```python
from build123d import *

# Parameters (mm, degrees)
BOSS_EXTRUDE1_DEPTH     = 250
BOSS_EXTRUDE2_DEPTH     = 50
SKETCH3_R               = 5
CUT_EXTRUDE1_DEPTH      = 319.801276513
FILLET1_R               = 10
MIRROR2_COPY_1_SKETCH_R = 5
MIRROR2_COPY_1_DEPTH    = 319.801276513
FILLET1_OF_MIRROR2_R    = 10
CUT_EXTRUDE2_DEPTH      = 282.035202699
FILLET2_R               = 25
CUT_EXTRUDE3_DEPTH      = 282.035202699
FILLET3_R               = 25
SKETCH6_R               = 5
CUT_EXTRUDE4_DEPTH      = 280.207367213
CUT_EXTRUDE5_DEPTH      = 170
FILLET4_R               = 10
FILLET5_R               = 25.875
FILLET6_R               = 10
BOSS_EXTRUDE3_DEPTH     = 30
SKETCH9_W               = 15.875
SKETCH9_H               = 40
BOSS_EXTRUDE4_DEPTH     = 140
FILLET7_R               = 25.875
FILLET8_R               = 10
SKETCH10_W              = 8.436021397
SKETCH10_H              = 40
CUT_EXTRUDE6_DEPTH      = 130
SKETCH11_R              = 5
CUT_EXTRUDE7_DEPTH      = 280.207367213


with BuildPart() as part:
    # Sketch1 → Boss-Extrude1 (new body)
    with BuildSketch(Plane.XY):
        Polygon((0, 0), (0, 110), (15.875, 110), (15.875, 0), (40, 0), (40, -70), (24.125, -70), (24.125, -15.875), (0, -15.875), align=None)
    extrude(amount=BOSS_EXTRUDE1_DEPTH)

    # Sketch2 → Boss-Extrude2 (add)
    with BuildSketch(Plane(origin=(0, 0, 0), x_dir=(-1, 0, 0), z_dir=(0, 0, -1))):
        Polygon((-32.0625, -70), (-82.0625, -70), (-82.0625, -77.9375), (17.9375, -77.9375), (17.9375, -70), align=None)
    boss_extrude2 = extrude(amount=-BOSS_EXTRUDE2_DEPTH)

    # Sketch3 → Cut-Extrude1 (cut, through all)
    with BuildSketch(Plane(origin=(0, -70, 0), x_dir=(1, 0, 0), z_dir=(0, 1, 0))):
        with Locations(Location((61.03125, -25, 0), (0, 0, 180))):
            Circle(SKETCH3_R)
    cut_extrude1 = extrude(amount=-CUT_EXTRUDE1_DEPTH, mode=Mode.SUBTRACT)

    # Mirror1: Cut-Extrude1 across plane
    add(cut_extrude1.mirror(Plane(origin=(32.0625, 0, 0), x_dir=(0, 0, 1), z_dir=(1, 0, 0))), mode=Mode.SUBTRACT)

    # Fillet1
    fillet1_edges = [part.edges().sort_by_distance(p)[0] for p in [
        (40, -70, 25),
        (24.125, -70, 25),
    ]]
    fillet(fillet1_edges, radius=FILLET1_R)

    # Mirror2: Boss-Extrude2, Cut-Extrude1 across plane
    add(boss_extrude2.mirror(Plane(origin=(0, 0, 125), x_dir=(1, 0, 0), z_dir=(0, 0, -1))))
    add(cut_extrude1.mirror(Plane(origin=(0, 0, 125), x_dir=(1, 0, 0), z_dir=(0, 0, -1))), mode=Mode.SUBTRACT)

    # Mirror2 copy 1 sketch → Mirror2 copy 1 (cut, through all)
    with BuildSketch(Plane(origin=(64.125, -70, 250), x_dir=(-1, 0, 0), z_dir=(0, 1, 0))):
        with Locations(Location((61.03125, -25, 0), (0, 0, 180))):
            Circle(MIRROR2_COPY_1_SKETCH_R)
    extrude(amount=-MIRROR2_COPY_1_DEPTH, mode=Mode.SUBTRACT)

    # Fillet1 of Mirror2
    fillet1_of_mirror2_edges = [part.edges().sort_by_distance(p)[0] for p in [
        (40, -70, 225),
        (24.125, -70, 225),
    ]]
    fillet(fillet1_of_mirror2_edges, radius=FILLET1_OF_MIRROR2_R)

    # Sketch4 → Cut-Extrude2 (cut, through all)
    with BuildSketch(Plane(origin=(15.875, 0, 0), x_dir=(0, 0, -1), z_dir=(1, 0, 0))):
        Polygon((0, 0), (-140, 0), (-140, 20), (-40, 20), (-40, 110), (0, 110), align=None)
    extrude(amount=-CUT_EXTRUDE2_DEPTH, mode=Mode.SUBTRACT)

    # Fillet2
    fillet2_edges = [part.edges().sort_by_distance(p)[0] for p in [
        (7.9375, 110, 40),
    ]]
    fillet(fillet2_edges, radius=FILLET2_R)

    # Sketch5 → Cut-Extrude3 (cut, through all)
    with BuildSketch(Plane(origin=(15.875, 0, 0), x_dir=(0, 0, -1), z_dir=(1, 0, 0))):
        Polygon((-250, 60), (-250, 110), (-200, 110), align=None)
    extrude(amount=-CUT_EXTRUDE3_DEPTH, mode=Mode.SUBTRACT)

    # Fillet3
    fillet3_edges = [part.edges().sort_by_distance(p)[0] for p in [
        (7.9375, 60, 250),
        (7.9375, 110, 200),
    ]]
    fillet(fillet3_edges, radius=FILLET3_R)

    # Sketch6 → Cut-Extrude4 (cut, through all)
    with BuildSketch(Plane(origin=(40, 0, 0), x_dir=(0, 0, -1), z_dir=(1, 0, 0))):
        with Locations((-65, 85)):
            Circle(SKETCH6_R)
        with Locations((-100, 85)):
            Circle(SKETCH6_R)
        with Locations((-128, 30)):
            Circle(SKETCH6_R)
        with Locations((-155, 20)):
            Circle(SKETCH6_R)
        with Locations(Location((-35, -25, 0), (0, 0, 90))):
            Circle(SKETCH6_R)
        with Locations(Location((-85, -25, 0), (0, 0, 90))):
            Circle(SKETCH6_R)
    extrude(amount=-CUT_EXTRUDE4_DEPTH, mode=Mode.SUBTRACT)

    # Sketch7 → Cut-Extrude5 (cut)
    with BuildSketch(Plane(origin=(0, 0, 0), x_dir=(-1, 0, 0), z_dir=(0, 0, -1))):
        Polygon((0, 0), (-40, 0), (-40, -40), (-24.125, -40), (-24.125, -15.875), (0, -15.875), align=None)
    extrude(amount=-CUT_EXTRUDE5_DEPTH, mode=Mode.SUBTRACT)

    # Fillet4
    fillet4_edges = [part.edges().sort_by_distance(p)[0] for p in [
        (7.9375, 20, 140),
    ]]
    fillet(fillet4_edges, radius=FILLET4_R)

    # Fillet5
    # the kernel refuses this fillet: 25.875 mm, written as the material it takes off along each edge
    with BuildSketch(Plane(origin=(40, 0, 105.460616433), x_dir=(-1, 0, 0), z_dir=(0, 0, 1))) as fillet5_piece_1:
        with BuildLine():
            CenterArc((25.875, 25.815753427), FILLET5_R, 180, 86.121962796)
            Line((0, 25.815753427), (-0.5175, 25.815753427))
            Line((-0.5175, 25.815753427), (-0.5175, 0))
            Line((-0.5175, 0), (0, -0.5175))
            ThreePointArc((0, -0.5175), (12.0625, -0.5175), (24.09, -0.516315069))
            Line((24.09, -0.516315069), (24.125, 0))
        make_face()
    extrude(amount=209.078767135, mode=Mode.SUBTRACT)

    # Fillet6
    fillet6_edges = [part.edges().sort_by_distance(p)[0] for p in [
        (15.875, 0, 210),
    ]]
    fillet(fillet6_edges, radius=FILLET6_R)

    # Sketch8 → Boss-Extrude3 (add)
    with BuildSketch(Plane(origin=(0, 0, 170), x_dir=(-1, 0, 0), z_dir=(0, 0, -1))):
        Polygon((-40, -40), (-24.125, -40), (-24.125, -15.875), (0, -15.875), (0, 0), (-40, 0), align=None)
    extrude(amount=BOSS_EXTRUDE3_DEPTH)

    # Sketch9 → Boss-Extrude4 (add)
    with BuildSketch(Plane(origin=(0, 0, 140), x_dir=(-1, 0, 0), z_dir=(0, 0, -1))):
        with Locations((-32.0625, -20)):
            Rectangle(SKETCH9_W, SKETCH9_H)
    extrude(amount=BOSS_EXTRUDE4_DEPTH)

    # Fillet7
    # the kernel refuses this fillet: 25.875 mm, written as the material it takes off along each edge
    with BuildSketch(Plane(origin=(0, -15.875, 75.460616433), x_dir=(1, 0, 0), z_dir=(0, 0, 1))) as fillet7_piece_1:
        with BuildLine():
            CenterArc((25.875, 25.815753427), FILLET7_R, 180, 86.121962796)
            Line((0, 25.815753427), (-0.5175, 25.815753427))
            Line((-0.5175, 25.815753427), (-0.5175, 0))
            Line((-0.5175, 0), (0, -0.5175))
            ThreePointArc((0, -0.5175), (12.0625, -0.5175), (24.09, -0.516315069))
            Line((24.09, -0.516315069), (24.125, 0))
        make_face()
    extrude(amount=239.078767135, mode=Mode.SUBTRACT)

    # Fillet8
    # the kernel refuses this fillet: 10 mm, written as the material it adds along each edge
    with BuildSketch(Plane(origin=(24.125, -15.875, 140), x_dir=(0, -1, 0), z_dir=(0, 0, 1))) as fillet8_piece_1:
        with BuildLine():
            CenterArc((8.080457645, -10), FILLET8_R, 90, 70.881309601)
            ThreePointArc((-1.36796356, -6.724738676), (-0.46005439, -3.407921221), (0, 0))
            Line((0, 0), (8.080457645, 0))
        make_face()
    extrude(amount=110)

    # Sketch10 → Cut-Extrude6 (cut)
    with BuildSketch(Plane(origin=(0, 0, 0), x_dir=(-1, 0, 0), z_dir=(0, 0, -1))):
        with Locations((-28.343010699, -20)):
            Rectangle(SKETCH10_W, SKETCH10_H)
    extrude(amount=-CUT_EXTRUDE6_DEPTH, mode=Mode.SUBTRACT)

    # Sketch11 → Cut-Extrude7 (cut, through all)
    with BuildSketch(Plane(origin=(40, 0, 0), x_dir=(0, 0, -1), z_dir=(1, 0, 0))):
        with Locations(Location((-35, -25, 0), (0, 0, 90))):
            Circle(SKETCH11_R)
        with Locations(Location((-85, -25, 0), (0, 0, 90))):
            Circle(SKETCH11_R)
    extrude(amount=-CUT_EXTRUDE7_DEPTH, mode=Mode.SUBTRACT)


solid = part.part
```
Geometry check sheet. Reference: the model listing, model coordinates, mm. A direction names the side the tool comes from. Give positions to 0.01 mm unless a question says otherwise; leave off trailing zeros. Order: outer loops, then holes, each group sorted by start corner. A loop starts at its lowest first (then second) coordinate and runs counter-clockwise, first axis right, second up. Notation, with made-up numbers: (-22.5, 2) - (-11.5, 2) arc R26 ccw to (-11.5, 32) - close; hole circle Ø6 at (32.5, -25). An arc over 180 degrees is marked (long way). Answer in a Markdown table with one row per item. Add a question column.
Q1. Cross-section at B-B, the plane x = -8. Enter the section's corners in (y, z), then the cut area to 3 significant figures.
Q2. Cross-section at C-C, the plane z = 35. Enter the section's corners in (x, y) (1 decimal).
Q3. Material ranges on probe 1 along Y at (x, z) = (9, 128); probe 2 along Y at (x, z) = (12.75, 65); probe 3 along X at (y, z) = (84, 152.5) (3 decimals), recorded low to high. Write a range as from..to.
Q4. Mould release check, pull along Z, two halves, no side actions. Record for faces 4 (the flat face through (8, 85, 225)), 5 (the flat face through (8, 110, 126)), 6 (the cylindrical face through (62.12, -73.91, 20.12)): pulls with the +Z half, pulls with the -Z half, needs draft (parallel to the pull), parting line crosses it, or undercut.
Q5. Cross-section at A-A, the plane z = 100. Enter the section's corners in (x, y) (3 decimals).
Q6. Cross-section at D-D, the plane y = -34. Enter the section's corners in (x, z) (3 decimals), then the cut area to 3 significant figures.
Q7. Tool access check on faces 1 (the cylindrical face through (4.665, -4.88, 194.23)), 2 (the flat face through (32.561, -20, 64)), 3 (the flat face through (34, -5, 170)). Record the directions out of +Z, -Z, +X, -X, +Y, -Y that give a thin tool (end or side, any length) a straight path to the whole face; none if there is none.
Q8. Gauge pin test, flat ends, axial feed: pin 1 (10 mm diameter, centred on x = -4, y = 76.5, fed in from -Z); pin 2 (13 mm diameter, centred on x = 61.03, z = 225, fed in from +Y); pin 3 (1.2 mm diameter, centred on x = 17, y = 2.5, fed in from -Z). Record the tip position at first contact, or that the pin passes through.
Check values:
| question | item | result |
|---|---|---|
| 1 | outline | (-77.94, 0) - (-70, 0) - (-70, 50) - (-77.94, 50) - close; (-77.94, 200) - (-70, 200) - (-70, 250) - (-77.94, 250) - close |
| 1 | area | 794 mm^2 |
| 2 | outline | (-17.9, -77.9) - (82.1, -77.9) - (82.1, -70) - (50, -70) arc R10 cw to (40, -60) - (40, -30) - (32.6, -30) - (32.6, -40) - (24.1, -40) - (24.1, -60) arc R10 cw to (14.1, -70) - (-17.9, -70) - close; (32.6, -20) - (40, -20) - (40, 0) - (32.6, 0) - close |
| 3 | probe 1 | y = 20..25, 35..110 |
| 3 | probe 2 | y = 20..80, 90..110 |
| 3 | probe 3 | x = 0..15.875 |
| 4 | face 4 | pulls with the +Z half |
| 4 | face 5 | needs draft |
| 4 | face 6 | undercut |
| 5 | outline | (0, 20) - (15.875, 20) - (15.875, 80) - (0, 80) - close; (0, 90) - (15.875, 90) - (15.875, 110) - (0, 110) - close; (24.125, -70) - (40, -70) - (40, 0) - (32.561, 0) - (32.561, -40) - (24.125, -40) - close |
| 6 | outline | (24.125, 130) - (32.561, 130) - (32.561, 0) - (40, 0) - (40, 250) - (24.125, 250) - close |
| 6 | area | 2,870 mm^2 |
| 7 | face 1 | +Z, -Z, -X |
| 7 | face 2 | -Z, -X, +Y |
| 7 | face 3 | +Z, +X, +Y |
| 8 | pin 1 | stops at z = 40 |
| 8 | pin 2 | stops at y = -70 |
| 8 | pin 3 | stops at z = 170 |
